Geometry: final body of the model. Coordinates: model frame, mm. Give positions to 0.01 mm unless a question says otherwise; leave off trailing zeros. Loops run counter-clockwise (first coordinate to the right, second up) from the corner with the lowest first, then second, coordinate; pieces in that order, holes last. Notation, with made-up numbers: (22.5, 29) - (69.5, 29) arc R22 ccw to (69.5, 60) - close; hole circle Ø7 at (-10.75, -14.75). An arc over 180 degrees is marked (long way). Answer in a Markdown table with one row per item.
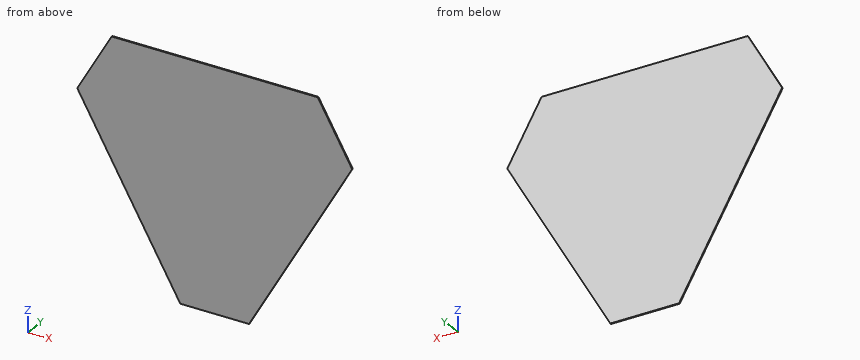
Autodesk Inventor part; units mm, degrees
ref_plane "YZ Plane" through (0, 0, 0) normal (1, 0, 0) x (0, 1, 0)
ref_plane "XZ Plane" through (0, 0, 0) normal (0, 1, 0) x (-1, 0, 0)
ref_plane "XY Plane" through (0, 0, 0) normal (0, 0, 1) x (1, 0, 0)
sketch "Sketch1" plane through (0, 0, 0) normal (0, 1, 0) x (-1, 0, 0)
  line L0 (304.8, 351.9527) -> (-304.8, 351.9527)
  line L1 (-304.8, 351.9527) -> (-406.4, 175.9764)
  line L2 (-406.4, 175.9764) -> (-101.6, -351.9527)
  line L3 (-101.6, -351.9527) -> (101.6, -351.9527)
  line L4 (101.6, -351.9527) -> (406.4, 175.9764)
  line L5 (406.4, 175.9764) -> (304.8, 351.9527)
  line L6 (-254, -87.9882) -> (0, 58.6588) construction
  line L7 (254, -87.9882) -> (0, 58.6588) construction
  line L8 (0, 351.9527) -> (0, 58.6588) construction
  point P0 (-355.6, 263.9645)
  dimension "d0" = 609.6
  dimension "d1" = 203.2
  dimension "d2" = 120
  dimension "d3" = 609.6
  dimension "d4" = 120
  dimension "d5" = 203.2
  dimension "d6" = 240
  dimension "d7" = 609.6
  dimension "d8" = 120
  dimension "d9" = 203.2
  dimension "d10" = 120
  dimension "d16" = 293.2939
  dimension "d17" = 120
  dimension "d18" = 120
  dimension "d19" = 120
extrude "Extrusion1" add sketch "Sketch1" against normal blind 3
properties part number "Top Plate"
Q1. First-contact query: pin 1 (1.5 mm diameter, centred on y = -1.5, z = -185.5, fed in from +X); pin 2 (1.5 mm diameter, centred on y = -1, z = -264.5, fed in from +X); pin 3 (1 mm diameter, centred on y = -0.5, z = -256.5, fed in from +X). Flat tips, straight axial feed; report the tip coordinate or a pass-through.
Check values:
| item | result |
|---|---|
| pin 1 | x = 198.13 |
| pin 2 | x = 152.52 |
| pin 3 | x = 157 |
Q2. Cut plane B-B (z = 143). Output: boundary loops of the cut face in (x, y).
Check values:
| item | result |
|---|---|
| outline | (-387.36, -3) - (387.36, -3) - (387.36, 0) - (-387.36, 0) - close |
Q3. Cut plane C-C (x = -252). Output: boundary loops of the cut face in (y, z).
Check values:
| item | result |
|---|---|
| outline | (-3, -91.45) - (0, -91.45) - (0, 351.95) - (-3, 351.95) - close |
Q4. Material intervals for line 1 along X through (y, z) = (-2.4, 227.5); line 2 along Z through (x, y) = (154, -1.65); line 3 along Z through (x, y) = (217, -1.9), sorted ascending.
Check values:
| item | result |
|---|---|
| line 1 | -376.65 to 376.65 |
| line 2 | -261.19 to 351.95 |
| line 3 | -152.07 to 351.95 |
Q5. Cut plane A-A (y = -2). Output: boundary loops of the cut face in (x, z).
Check values:
| item | result |
|---|---|
| outline | (-406.4, 175.98) - (-101.6, -351.95) - (101.6, -351.95) - (406.4, 175.98) - (304.8, 351.95) - (-304.8, 351.95) - close |
